from build123d import *

# Parameters (mm, degrees)
EXTRUDE_1_DEPTH      = 10
SKETCH_2_R           = 2.5
CUT_EXTRUDE_1_DEPTH  = 10
CHAMFER_1_SIZE       = 2
SKETCH_4_R           = 22.5
CUT_EXTRUDE_3_DEPTH  = 36
SKETCH_9_R           = 3
CUT_EXTRUDE_8_DEPTH  = 13
SKETCH_10_R          = 4.25
CUT_EXTRUDE_9_DEPTH  = 13
CHAMFER_6_SIZE       = 1
SKETCH_6_R           = 7.5
CUT_EXTRUDE_10_DEPTH = 10
SKETCH_11_R          = 2
CUT_EXTRUDE_11_DEPTH = 15
SKETCH_12_R          = 2
CUT_EXTRUDE_12_DEPTH = 15
SKETCH_13_R          = 2
CUT_EXTRUDE_13_DEPTH = 10
SKETCH_14_R          = 22.5
SKETCH_14_R_2        = 4.25
SKETCH_14_R_3        = 2.5
SKETCH_14_R_4        = 3
SKETCH_14_R_5        = 2
SKETCH_14_R_6        = 7.5
EXTRUDE_2_DEPTH      = 10
CHAMFER_7_SIZE       = 2.9
CHAMFER_8_SIZE       = 1.9
FILLET_2_R           = 3


with BuildPart() as part:
    # Эскиз1 → Бобышка-Вытянуть1 (new body)
    with BuildSketch(Plane(origin=(0, 0, 0), x_dir=(1, 0, 0), z_dir=(0, 1, 0))):
        with BuildLine():
            Line((-172.682149641, 42.5), (-12.334194433, 42.5))
            ThreePointArc((-12.334194433, 42.5), (74.978715977, 0), (-12.334194433, -42.5))
            Line((-12.334194433, -42.5), (-172.682149641, -42.5))
            ThreePointArc((-172.682149641, -42.5), (-249.021284023, 0), (-172.682149641, 42.5))
        make_face()
    extrude(amount=EXTRUDE_1_DEPTH)

    # Эскиз2 → Вырез-Вытянуть1 (cut)
    with BuildSketch(Plane(origin=(0, 10, 0), x_dir=(1, 0, 0), z_dir=(0, 1, 0))):
        with Locations(Location((20.978715977, 31.5, 0), (0, 0, 270))):
            Circle(SKETCH_2_R)
        with Locations(Location((-10.521284023, 0, 0), (0, 0, 270))):
            Circle(SKETCH_2_R)
        with Locations(Location((20.978715977, -31.5, 0), (0, 0, 270))):
            Circle(SKETCH_2_R)
        with Locations(Location((52.478715977, 0, 0), (0, 0, 270))):
            Circle(SKETCH_2_R)
    extrude(amount=-CUT_EXTRUDE_1_DEPTH, mode=Mode.SUBTRACT)

    # Фаска1
    chamfer_1_edges = [part.edges().sort_by_distance(p)[0] for p in [
        (20.978715977, 0, -34),
        (-10.521284023, 0, -2.5),
        (20.978715977, 0, 29),
        (52.478715977, 0, -2.5),
    ]]
    chamfer(chamfer_1_edges, length=CHAMFER_1_SIZE)

    # Эскиз4 → Вырез-Вытянуть3 (cut)
    with BuildSketch(Plane.XZ):
        with Locations(Location((20.978715977, 0, 0), (0, 0, 270))):
            Circle(SKETCH_4_R)
    extrude(amount=-CUT_EXTRUDE_3_DEPTH, mode=Mode.SUBTRACT)

    # Эскиз9 → Вырез-Вытянуть8 (cut)
    with BuildSketch(Plane(origin=(0, 10, 0), x_dir=(1, 0, 0), z_dir=(0, 1, 0))):
        with Locations(Location((-39.951971169, 0, 0), (0, 0, 270))):
            Circle(SKETCH_9_R)
    extrude(amount=-CUT_EXTRUDE_8_DEPTH, mode=Mode.SUBTRACT)

    # Эскиз10 → Вырез-Вытянуть9 (cut)
    with BuildSketch(Plane(origin=(0, 10, 0), x_dir=(1, 0, 0), z_dir=(0, 1, 0))):
        with Locations(Location((-37.333322344, 18.054624514, 0), (0, 0, 270))):
            Circle(SKETCH_10_R)
    extrude(amount=-CUT_EXTRUDE_9_DEPTH, mode=Mode.SUBTRACT)

    # Фаска6
    chamfer_6_edges = [part.edges().sort_by_distance(p)[0] for p in [
        (-37.333322344, 0, -22.304624514),
    ]]
    chamfer(chamfer_6_edges, length=CHAMFER_6_SIZE)

    # Эскиз6 → Вырез-Вытянуть10 (cut)
    with BuildSketch(Plane.XZ):
        with Locations(Location((-209.021284023, 0, 0), (0, 0, 270))):
            Circle(SKETCH_6_R)
    extrude(amount=-CUT_EXTRUDE_10_DEPTH, mode=Mode.SUBTRACT)

    # Эскиз11 → Вырез-Вытянуть11 (cut)
    with BuildSketch(Plane.XZ):
        with Locations(Location((-117.021284023, 24, 0), (0, 0, 270))):
            Circle(SKETCH_11_R)
        with Locations(Location((-117.021284023, -24, 0), (0, 0, 270))):
            Circle(SKETCH_11_R)
    extrude(amount=-CUT_EXTRUDE_11_DEPTH, mode=Mode.SUBTRACT)

    # Эскиз12 → Вырез-Вытянуть12 (cut)
    with BuildSketch(Plane.XZ):
        with Locations(Location((-151.021284023, 0, 0), (0, 0, 270))):
            Circle(SKETCH_12_R)
        with Locations(Location((-132.021284023, 0, 0), (0, 0, 270))):
            Circle(SKETCH_12_R)
    extrude(amount=-CUT_EXTRUDE_12_DEPTH, mode=Mode.SUBTRACT)

    # Эскиз13 → Вырез-Вытянуть13 (cut)
    with BuildSketch(Plane(origin=(0, 0, 0), x_dir=(-1, 0, 0), z_dir=(0, -1, 0))):
        with Locations(Location((219.627885741, -10.606601718, 0), (0, 0, 90))):
            Circle(SKETCH_13_R)
        with Locations(Location((198.414682305, -10.606601718, 0), (0, 0, 90))):
            Circle(SKETCH_13_R)
        with Locations(Location((219.627885741, 10.606601718, 0), (0, 0, 90))):
            Circle(SKETCH_13_R)
        with Locations(Location((198.414682305, 10.606601718, 0), (0, 0, 90))):
            Circle(SKETCH_13_R)
    extrude(amount=-CUT_EXTRUDE_13_DEPTH, mode=Mode.SUBTRACT)

    # Эскиз14 → Бобышка-Вытянуть2 (add)
    with BuildSketch(Plane(origin=(0, 0, 0), x_dir=(-1, 0, 0), z_dir=(0, -1, 0))):
        Polygon((170.810605904, -42.5), (12.888816391, -42.5), (1.388816391, -54), (-43.346248345, -54), (-74.978715977, -22.367532368), (-74.978715977, 22.367532368), (-43.346248345, 54), (1.388816391, 54), (12.888816391, 42.5), (170.810605904, 42.5), (178.310605904, 50), (219.731962142, 50), (249.021284023, 20.710678119), (249.021284023, -20.710678119), (219.731962142, -50), (178.310605904, -50), align=None)
        with Locations(Location((-20.978715977, 0, 0), (0, 0, 90))):
            Circle(SKETCH_14_R, mode=Mode.SUBTRACT)
        with Locations(Location((37.333322344, 18.054624514, 0), (0, 0, 270))):
            Circle(SKETCH_14_R_2, mode=Mode.SUBTRACT)
        with Locations(Location((10.521284023, 0, 0), (0, 0, 270))):
            Circle(SKETCH_14_R_3, mode=Mode.SUBTRACT)
        with Locations(Location((-52.478715977, 0, 0), (0, 0, 270))):
            Circle(SKETCH_14_R_3, mode=Mode.SUBTRACT)
        with Locations(Location((-20.978715977, 31.5, 0), (0, 0, 270))):
            Circle(SKETCH_14_R_3, mode=Mode.SUBTRACT)
        with Locations(Location((-20.978715977, -31.5, 0), (0, 0, 270))):
            Circle(SKETCH_14_R_3, mode=Mode.SUBTRACT)
        with Locations(Location((39.951971169, 0, 0), (0, 0, 270))):
            Circle(SKETCH_14_R_4, mode=Mode.SUBTRACT)
        with Locations(Location((117.021284023, 24, 0), (0, 0, 90))):
            Circle(SKETCH_14_R_5, mode=Mode.SUBTRACT)
        with Locations(Location((132.021284023, 0, 0), (0, 0, 90))):
            Circle(SKETCH_14_R_5, mode=Mode.SUBTRACT)
        with Locations(Location((117.021284023, -24, 0), (0, 0, 90))):
            Circle(SKETCH_14_R_5, mode=Mode.SUBTRACT)
        with Locations(Location((151.021284023, 0, 0), (0, 0, 90))):
            Circle(SKETCH_14_R_5, mode=Mode.SUBTRACT)
        with Locations(Location((198.414682305, -10.606601718, 0), (0, 0, 90))):
            Circle(SKETCH_14_R_5, mode=Mode.SUBTRACT)
        with Locations(Location((198.414682305, 10.606601718, 0), (0, 0, 90))):
            Circle(SKETCH_14_R_5, mode=Mode.SUBTRACT)
        with Locations(Location((209.021284023, 0, 0), (0, 0, 90))):
            Circle(SKETCH_14_R_6, mode=Mode.SUBTRACT)
        with Locations(Location((219.627885741, 10.606601718, 0), (0, 0, 90))):
            Circle(SKETCH_14_R_5, mode=Mode.SUBTRACT)
        with Locations(Location((219.627885741, -10.606601718, 0), (0, 0, 90))):
            Circle(SKETCH_14_R_5, mode=Mode.SUBTRACT)
    extrude(amount=-EXTRUDE_2_DEPTH)

    # Фаска7
    chamfer_7_edges = [part.edges().sort_by_distance(p)[0] for p in [
        (-10.521284023, 0, -2.5),
        (52.478715977, 0, -2.5),
        (20.978715977, 0, -34),
        (20.978715977, 0, 29),
    ]]
    chamfer(chamfer_7_edges, length=CHAMFER_7_SIZE)

    # Фаска8
    chamfer_8_edges = [part.edges().sort_by_distance(p)[0] for p in [
        (-198.414682305, 0, 12.606601718),
        (-219.627885741, 0, -8.606601718),
        (-198.414682305, 0, -8.606601718),
        (-219.627885741, 0, 12.606601718),
    ]]
    chamfer(chamfer_8_edges, length=CHAMFER_8_SIZE)

    # Скругление2
    fillet_2_edges = [part.edges().sort_by_distance(p)[0] for p in [
        (-170.810605904, 5, 42.5),
        (-12.888816391, 5, 42.5),
        (-12.888816391, 5, -42.5),
        (-170.810605904, 5, -42.5),
    ]]
    fillet(fillet_2_edges, radius=FILLET_2_R)


solid = part.part
Model file for the job. Use its own axes, mm. A direction names the side the tool comes from. Give positions to 0.01 mm unless a question says otherwise; leave off trailing zeros. Order: outer loops, then holes, each group sorted by start corner. A loop starts at its lowest first (then second) coordinate and runs counter-clockwise, first axis right, second up. Notation, with made-up numbers: (0.5, 12) - (45.5, 12) arc R13 ccw to (45.5, 31) - close; hole circle Ø3 at (-1, 18). An arc over 180 degrees is marked (long way). Write item = value, one per line. Start each with the question number.
1. Cut at A-A, the plane x = -74. List the corners of the cut face in (y, z).
2. Drop flat-ended pins along their axis: P1, Ø4, axis at x = -101, y = 9, coming from the +Z side; P2, Ø3.5, axis at x = -198.41, z = 10.61, coming from the -Y side; P3, Ø5, axis at y = 5, z = 33.5, coming from the -X side; P4, Ø1.5, axis at x = -17, y = 8.5, coming from the -Z side. Give the stop position or say it passes through.
3. Cut at B-B, the plane y = 4.5. State how many separate pieces and enclosed holes the cut face has, and give its area (3 significant figures).
4. Probe line 1 along Z through (x, y) = (-192, 5.5); line 2 along X through (y, z) = (8.25, -48); line 3 along X through (y, z) = (9, -16). List the from-to ranges inside material, lowest first.
5. Which spindle directions (+Z, -Z, +X, -X, +Y, -Y) get a long thin tool onto all of the face, cutting with end or side? Do faces 1 (the cylindrical face through (43.287, 4.93, 2.929)), 2 (the flat face through (-6.774, 4.93, 48.615)), 3 (the flat face through (-199, 5, -50)). Say none if no direction does.
6. Two-plate mould, pull along Z, no slides. Class faces 4 (the flat face through (-249.021, 5, 0)), 5 (the cylindrical face through (-216.34, 4.93, 1.63)), 6 (the flat face through (-199, 5, 50)): pulls with the +Z half, pulls with the -Z half, needs draft (parallel to the pull), parting line crosses it, or undercut.
Taken from the geometry:
q1.outline = (0, -42.5) - (10, -42.5) - (10, 42.5) - (0, 42.5) - close
q2.P1 = 42.5
q2.P2 = through
q2.P3 = -238.73
q2.P4 = -42.5
q3.separate_pieces = 1
q3.enclosed_holes = 16
q3.area = 26,700 mm²
q4.line_1 = -50 to 50
q4.line_2 = -221.73 to -176.31, -7.39 to 49.35
q4.line_3 = -249.02 to -41.05, -33.61 to 5.16, 36.8 to 74.98
q5.face_1 = +Y, -Y
q5.face_2 = +Z, +Y, -Y
q5.face_3 = -Z, -X, +Y, -Y
q6.face_4 = needs draft
q6.face_5 = undercut
q6.face_6 = pulls with the +Z half
